```python
from build123d import *

# Parameters (mm, degrees)
F1_DEPTH = 25.4
F2_R     = 5.08
F3_W     = 25.4
F3_H     = 17.4376570841
F4_DEPTH = 25.4
F5_W     = 17.797825551
F5_H     = 19.2676950246
F6_DEPTH = 25.4
F7_R     = 5.08


with BuildPart() as f1:
    # F0 (on Right) → F1 (new body)
    with BuildSketch(Plane.YZ):
        Polygon((136.5167200565, 44.1473908722), (81.1095386744, 44.2778617144), (61.5900829434, 51.9239269197), (48.8699753419, 19.451070548), (99.5989143848, 19.451070548), (99.5989143848, 0), (136.5167200565, 0), align=None)
    extrude(amount=F1_DEPTH)

    # F2
    f2_edges = [f1.edges().sort_by_distance(p)[0] for p in [
        (12.7, 99.598914, 19.451071),
    ]]
    fillet(f2_edges, radius=F2_R)

    # F3 (on face) → F4 (join)
    with BuildSketch(Plane(origin=(0, 35.7631713916, -14.0089736199), x_dir=(1, 0, 0), z_dir=(0, -0.9311129418, 0.3647309825))):
        with Locations((12.7, 44.6543661825)):
            Rectangle(F3_W, F3_H)
    extrude(amount=F4_DEPTH)

    # F5 (on face) → F6 (join)
    with BuildSketch(Plane(origin=(0, 136.5167200565, 0), x_dir=(-1, 0, 0), z_dir=(0, 1, 0))):
        with Locations((-34.2989127755, 9.6338475123)):
            Rectangle(F5_W, F5_H)
    extrude(amount=-F6_DEPTH)

    # F7
    f7_edges = [f1.edges().sort_by_distance(p)[0] for p in [
        (25.4, 123.81672, 19.267695),
    ]]
    fillet(f7_edges, radius=F7_R)


solid = f1.part
```
Geometry check sheet. Reference: the model listing, model coordinates, mm. A direction names the side the tool comes from. Give positions to 0.01 mm unless a question says otherwise; leave off trailing zeros. Order: outer loops, then holes, each group sorted by start corner. A loop starts at its lowest first (then second) coordinate and runs counter-clockwise, first axis right, second up. Notation, with made-up numbers: (44, 37) - (52, 37) arc R27 cw to (52, 55) - close; hole circle Ø7 at (56, -1.5). An arc over 180 degrees is marked (long way). Answer in a Markdown table with one row per item. Add a question column.
Q1. Cross-section at B-B, the plane x = 4.5. Enter the section's corners in (y, z), then the cut area to 3 significant figures.
Q2. Mould release check, pull along Y, two halves, no side actions. Record for faces 6 (the flat face through (22, 122, 0)), 7 (the flat face through (12.52, 37.21, 24.02)), 8 (the flat face through (12.522, 43.57, 40.255)), 9 (the flat face through (12.522, 58.455, 43.919)): pulls with the +Y half, pulls with the -Y half, needs draft (parallel to the pull), parting line crosses it, or undercut.
Q3. Tool access check on faces 1 (the flat face through (43.198, 124, 9)), 2 (the flat face through (13, 71, 19.451)), 3 (the flat face through (25.4, 83, 29)), 4 (the flat face through (34, 111.117, 10)), 5 (the flat face through (37, 124, 19.268)). Record the directions out of +Z, -Z, +X, -X, +Y, -Y that give a thin tool (end or side, any length) a straight path to the whole face; none if there is none.
Q4. Cross-section at D-D, the plane x = 37. Enter the section's corners in (y, z).
Q5. Cross-section at A-A, the plane z = 5. Enter the section's corners in (x, y).
Q6. Cross-section at C-C, the plane y = 114.5. Enter the section's corners in (x, z), then the cut area to 3 significant figures.
Q7. Gauge pin test, flat ends, axial feed: pin 1 (5 mm diameter, centred on x = 26.5, y = 108, fed in from +Z); pin 2 (7 mm diameter, centred on x = 15, z = 5.5, fed in from -Y); pin 3 (12.5 mm diameter, centred on x = 11.5, y = 75, fed in from -Z); pin 4 (3 mm diameter, centred on y = 123, z = 21.5, fed in from -X). Record the tip position at first contact, or that the pin passes through.
Q8. Material ranges on probe 1 along Z at (x, y) = (5, 128); probe 2 along X at (y, z) = (78, 44); probe 3 along Y at (x, z) = (41.5, 9), recorded low to high. Write a range as from..to.
Check values:
| question | item | result |
|---|---|---|
| 1 | outline | (25.22, 28.72) - (48.87, 19.45) - (94.52, 19.45) arc R5.08 cw to (99.6, 14.37) - (99.6, 0) - (136.52, 0) - (136.52, 44.15) - (81.11, 44.28) - (61.59, 51.92) - (55.23, 35.69) - (31.58, 44.95) - close |
| 1 | area | 3,300 mm^2 |
| 2 | face 6 | needs draft |
| 2 | face 7 | pulls with the -Y half |
| 2 | face 8 | undercut |
| 2 | face 9 | undercut |
| 3 | face 1 | +Z, -Z, +X, +Y, -Y |
| 3 | face 2 | -Z, +X, -X, -Y |
| 3 | face 3 | +Z, +X, -Y |
| 3 | face 4 | +Z, -Z, +X, -Y |
| 3 | face 5 | +Z, +X, +Y, -Y |
| 4 | outline | (111.12, 0) - (136.52, 0) - (136.52, 19.27) - (111.12, 19.27) - close |
| 5 | outline | (0, 99.6) - (25.4, 99.6) - (25.4, 111.12) - (43.2, 111.12) - (43.2, 136.52) - (0, 136.52) - close |
| 6 | outline | (0, 0) - (43.2, 0) - (43.2, 19.27) - (30.48, 19.27) arc R5.08 cw to (25.4, 24.35) - (25.4, 44.2) - (0, 44.2) - close |
| 6 | area | 1,470 mm^2 |
| 7 | pin 1 | stops at z = 44.22 |
| 7 | pin 2 | stops at y = 99.6 |
| 7 | pin 3 | stops at z = 19.45 |
| 7 | pin 4 | stops at x = 0 |
| 8 | probe 1 | z = 0..44.17 |
| 8 | probe 2 | x = 0..25.4 |
| 8 | probe 3 | y = 111.12..136.52 |
